Design review of the part built by this model. Coordinates are the model's own, in mm. Face numbers are marked on the shaded views. A direction names the side the tool comes from. Give positions to 0.01 mm unless a question says otherwise; leave off trailing zeros. Write each loop counter-clockwise with the first axis right and the second up, starting at its lowest first coordinate (ties: lowest second). Pieces come first, ordered by that corner, then holes. Notation, with made-up numbers: (59, 44.25) -> (67, 44.25) arc R14 cw to (67, 66.25) -> close; hole circle Ø10 at (77, 88). An arc over 180 degrees is marked (long way). Answer as a JSON object with one key per item and string values.
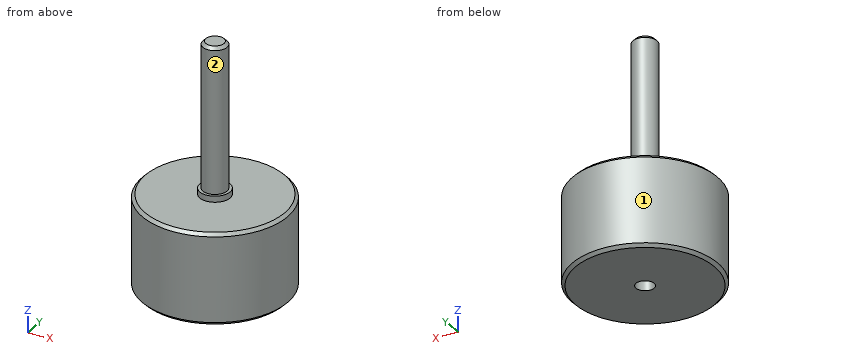
```python
from build123d import *

# Parameters (mm, degrees)
ESQUISSE1_R             = 24
BOSS_EXTRU_1_DEPTH      = 30
ESQUISSE2_R             = 4
BOSS_EXTRU_2_DEPTH      = 50
ESQUISSE3_R             = 5
BOSS_EXTRU_3_DEPTH      = 2
ESQUISSE4_R             = 3
ENL_V_MAT_EXTRU_1_DEPTH = 10
CHANFREIN1_SIZE         = 1


with BuildPart() as part:
    # Esquisse1 → Boss.-Extru.1 (new body)
    with BuildSketch(Plane.XY):
        Circle(ESQUISSE1_R)
    extrude(amount=BOSS_EXTRU_1_DEPTH)

    # Esquisse2 → Boss.-Extru.2 (add)
    with BuildSketch(Plane.XY.offset(30)):
        Circle(ESQUISSE2_R)
    extrude(amount=BOSS_EXTRU_2_DEPTH)

    # Esquisse3 → Boss.-Extru.3 (add)
    with BuildSketch(Plane.XY.offset(30)):
        Circle(ESQUISSE3_R)
    extrude(amount=BOSS_EXTRU_3_DEPTH)

    # Esquisse4 → Enlèv. mat.-Extru.1 (cut)
    with BuildSketch(Plane(origin=(0, 0, 0), x_dir=(-1, 0, 0), z_dir=(0, 0, -1))):
        Circle(ESQUISSE4_R)
    extrude(amount=-ENL_V_MAT_EXTRU_1_DEPTH, mode=Mode.SUBTRACT)

    # Chanfrein1
    chanfrein1_edges = [part.edges().sort_by_distance(p)[0] for p in [
        (-24, 0, 0),
        (-24, 0, 30),
        (-4, 0, 80),
    ]]
    chamfer(chanfrein1_edges, length=CHANFREIN1_SIZE)


solid = part.part
```
(1) For line 1 along Y through (x, z) = (0, 3.75); line 2 along Z through (x, y) = (-6, -9); line 3 along X through (y, z) = (0, 56), list the stretches that pass through material, from the lowest coordinate up.
Here are the results:
{"line 1": "y = -24 to -3, 3 to 24", "line 2": "z = 0 to 30", "line 3": "x = -4 to 4"}
(2) Clearance check with flat-ended pins moving along their axes: pin 1 (4 mm diameter, centred on x = 5.5, y = -10.5, fed in from +Z); pin 2 (3 mm diameter, centred on x = -18.5, z = 32.5, fed in from -Y); pin 3 (5.5 mm diameter, centred on x = 0, y = 0, fed in from -Z); pin 4 (8 mm diameter, centred on y = -8.5, z = 9, fed in from +X). State where each tip first meets the part, or that it passes through.
Here are the results:
{"pin 1": "stops at z = 30", "pin 2": "passes through", "pin 3": "stops at z = 10", "pin 4": "stops at x = 23.57"}
(3) For the marked faces 1 and 2, list the 3-axis set-ups (+Z, -Z, +X, -X, +Y, -Y) from which the entire face can be reached by the end or side of a thin tool; tool diameter is ignored.
Here are the results:
{"face 1": "+Z, -Z", "face 2": "+Z"}
(4) We need section C-C, the plane z = 27. State the section outline as (x, y) points.
Here are the results:
{"outline": "circle Ø48 at (0, 0)"}
(5) We need section D-D, the plane z = 62.5. State the section outline as (x, y) points, then the cut area to 3 significant figures.
Here are the results:
{"outline": "circle Ø8 at (0, 0)", "area": "50.3 mm²"}
(6) We need section A-A, the plane y = 0. State the section outline as (x, z) points.
Here are the results:
{"outline": "(-24, 1) -> (-23, 0) -> (-3, 0) -> (-3, 10) -> (3, 10) -> (3, 0) -> (23, 0) -> (24, 1) -> (24, 29) -> (23, 30) -> (5, 30) -> (5, 32) -> (4, 32) -> (4, 79) -> (3, 80) -> (-3, 80) -> (-4, 79) -> (-4, 32) -> (-5, 32) -> (-5, 30) -> (-23, 30) -> (-24, 29) -> close"}
